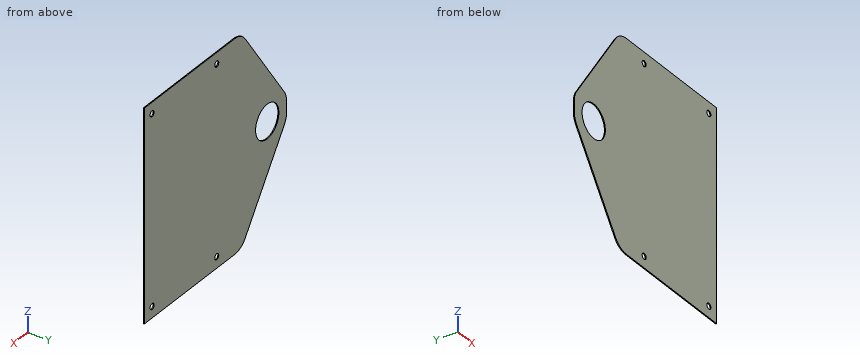
Autodesk Inventor part; units mm, degrees
ref_plane "YZ Plane" through (0, 0, 0) normal (1, 0, 0) x (0, 1, 0)
ref_plane "XZ Plane" through (0, 0, 0) normal (0, 1, 0) x (-1, 0, 0)
ref_plane "XY Plane" through (0, 0, 0) normal (0, 0, 1) x (1, 0, 0)
sketch "Sketch2" plane through (0, 0, 0) normal (0, 1, 0) x (-1, 0, 0)
  line L0 (0, 0) -> (69.7934, 0)
  line L1 (110, -53.1522) -> (110, -58.8478)
  line L2 (69.7934, -112) -> (0, -112)
  line L3 (0, -112) -> (0, 0)
  line L4 (77.9858, -4.2654) -> (108.1923, -47.4176)
  line L5 (77.9858, -107.7346) -> (108.1923, -64.5824)
  arc A0 (110, -53.1522) -> (108.1923, -47.4176) centre (100, -53.1522) ccw
  arc A1 (108.1923, -64.5824) -> (110, -58.8478) centre (100, -58.8478) ccw
  arc A2 (77.9858, -4.2654) -> (69.7934, 0) centre (69.7934, -10) ccw
  arc A3 (69.7934, -112) -> (77.9858, -107.7346) centre (69.7934, -102) ccw
  point P0 (110, -112)
  point P1 (110, 0)
  point P2 (75, 0)
  point P3 (110, -50)
  point P4 (75, -112)
  point P5 (110, -62)
  dimension "d10" = 110
  dimension "d11" = 112
  dimension "d34" = 35
  dimension "d35" = 50
  dimension "d36" = 35
  dimension "d37" = 50
  dimension "d38" = 10
extrude "Plate1" add sketch "Sketch2" along normal blind 0.5
sketch "Sketch3" plane through (0, 0.5, 0) normal (0, 1, 0) x (1, 0, 0)
  line L0 (0, 0) -> (-69.7934, 0)
  line L1 (-69.7934, 112) -> (0, 112)
  line L2 (0, 112) -> (0, 0)
  circle A0 centre (-6, 6) radius 1.55
  line L3 (0, 59.1522) -> (-110, 59.1522) construction
  line L4 (-110, 53.1522) -> (-110, 58.8478)
  line L5 (-6, 0) -> (-6, 112) construction
  circle A1 centre (-6, 106) radius 1.55
  circle A2 centre (-56, 6) radius 1.55
  circle A3 centre (-56, 106) radius 1.55
  point P0 (-62, 0)
  point P1 (-62, 112)
  point P2 (-110, 58.8478)
  dimension "d16" = 3.1
  dimension "d17" = 6
  dimension "d18" = 6
  dimension "d21" = 100
  dimension "d24" = 50
hole "Hole1" at (-56, 0.5, -6) at (-6, 0.5, -6) at (-6, 0.5, -106) at (-56, 0.5, -106) direction (0, -1, 0) diameter 3.1 end through all
sketch "Sketch4" plane through (0, 0.5, 0) normal (0, 1, 0) x (1, 0, 0)
  circle A0 centre (-56, 6) radius 1.55
  circle A1 centre (-56, 106) radius 1.55
  line L0 (-56, 6) -> (-56, 106) construction
  line L1 (-56, 106) -> (-56, 56)
  line L2 (-56, 56) -> (-110, 56) construction
  line L3 (-110, 53.1522) -> (-110, 58.8478)
  circle A2 centre (-95, 56) radius 9
  line L4 (-110, 53.1522) -> (-110, 58.8478)
  point P0 (0, 0)
  dimension "d39" = 18
  dimension "d40" = 15
hole "Hole2" at (-95, 0.5, -56) direction (0, -1, 0) diameter 18 end through all
equation "\"d32\" = Thickness"
equation "\"BendRadius\" = Thickness"
equation "\"BendReliefWidth\" = Thickness"
equation "\"BendReliefDepth\" = 0.5 * Thickness"
equation "\"CornerReliefSize\" = 4 * Thickness"
equation "\"MinimumRemnant\" = 2 * Thickness"
equation "\"TransitionRadius\" = BendRadius"
equation "\"JacobiRadiusSize\" = BendRadius"
equation "\"GapSize\" = Thickness"
properties part number "Sketch-3-44"
Read the model definition and answer for the solid it produces. Units are mm, in the model's axes. Coordinates: 2 decimals unless noted, no trailing zeros. Write each loop counter-clockwise with the first axis right and the second up, starting at its lowest first coordinate (ties: lowest second). Pieces come first, ordered by that corner, then holes. Notation, with made-up numbers: (50.25, 7.5) -> (85.25, 7.5) arc R25 ccw to (85.25, 44.5) -> close; hole circle Ø1 at (3.5, 89.25). An arc over 180 degrees is marked (long way). Write item = value, one per line.
(1) Section A-A on x = -6 is taken. Write down the section's boundary in (y, z).
From the geometry:
outline = (0, -112) -> (0.5, -112) -> (0.5, -107.55) -> (0, -107.55) -> close; (0, -104.45) -> (0.5, -104.45) -> (0.5, -7.55) -> (0, -7.55) -> close; (0, -4.45) -> (0.5, -4.45) -> (0.5, 0) -> (0, 0) -> close
(2) Section D-D on x = -101.5 is taken. Write down the section's boundary in (y, z).
From the geometry:
outline = (0, -74.14) -> (0.5, -74.14) -> (0.5, -62.22) -> (0, -62.22) -> close; (0, -49.78) -> (0.5, -49.78) -> (0.5, -37.86) -> (0, -37.86) -> close
(3) Given pin 1 Ø2.5 at (x, z) = (-56, -106) entering from -Y, flat-ended and moving along its own axis, determine where the tip first touches the part or whether it passes through.
From the geometry:
pin_1 = through
(4) Section C-C on y = 0.35 is taken. Write down the section's boundary in (x, z).
From the geometry:
outline = (-110, -58.85) arc R10 ccw to (-108.19, -64.58) -> (-77.99, -107.73) arc R10 ccw to (-69.79, -112) -> (0, -112) -> (0, 0) -> (-69.79, 0) arc R10 ccw to (-77.99, -4.27) -> (-108.19, -47.42) arc R10 ccw to (-110, -53.15) -> close; hole circle Ø18 at (-95, -56); hole circle Ø3.1 at (-56, -106); hole circle Ø3.1 at (-56, -6); hole circle Ø3.1 at (-6, -106); hole circle Ø3.1 at (-6, -6)
(5) Section B-B on z = -56 is taken. Write down the section's boundary in (x, y).
From the geometry:
outline = (-110, 0) -> (-104, 0) -> (-104, 0.5) -> (-110, 0.5) -> close; (-86, 0) -> (0, 0) -> (0, 0.5) -> (-86, 0.5) -> close
(6) Straight lines are drawn through the part: L1, parallel to Z at x = -56, y = 0.4; L2, parallel to X at y = 0.1, z = -56; L3, parallel to X at y = 0.4, z = -6. For each, find the intervals that lie inside material, in ascending order. Write a range as from..to.
From the geometry:
L1 = -112..-107.55, -104.45..-7.55, -4.45..0
L2 = -110..-104, -86..0
L3 = -79.2..-57.55, -54.45..-7.55, -4.45..0
